from build123d import *

# Parameters (mm, degrees)
EXTRUDE_1_DEPTH      = 10
SKETCH_5_R           = 2.6
CUT_EXTRUDE_3_DEPTH  = 10
FILLET_5_R           = 3
FILLET_6_R           = 3
FILLET_7_R           = 3
SKETCH_7_R           = 5.5
CUT_EXTRUDE_4_DEPTH  = 5
SKETCH_12_R          = 2.553682631
CUT_EXTRUDE_9_DEPTH  = 9
EXTRUDE_2_DEPTH      = 5
CUT_EXTRUDE_START    = 5
SKETCH_14_R          = 5.5
CUT_EXTRUDE_12_DEPTH = 5
EXTRUDE_START        = 5
EXTRUDE_6_DEPTH      = 5
SKETCH_22_R          = 5.5
EXTRUDE_7_DEPTH      = 5
SKETCH_24_R          = 5.5
CUT_EXTRUDE_14_DEPTH = 3
SKETCH_25_R          = 2.65
CUT_EXTRUDE_15_DEPTH = 3
SKETCH_26_R          = 2.65
CUT_EXTRUDE_16_DEPTH = 5
SKETCH_29_R          = 2.65
EXTRUDE_8_DEPTH      = 10
EXTRUDE_START_2      = 3
SKETCH_30_R          = 5.5
EXTRUDE_9_DEPTH      = 3
CUT_EXTRUDE_18_DEPTH = 3
SKETCH_33_R          = 5.5
SKETCH_33_R_2        = 2.6
EXTRUDE_10_DEPTH     = 5
SKETCH_34_W          = 118.655960463
SKETCH_34_H          = 108.474675719
CUT_EXTRUDE_20_DEPTH = 3
CUT_EXTRUDE_21_DEPTH = 108.211729676


with BuildPart() as part:
    # 草图1 → 凸台-拉伸1 (new body)
    with BuildSketch(Plane(origin=(0, 0, 0), x_dir=(1, 0, 0), z_dir=(0, 1, 0))):
        Polygon((0, 0), (0, 80), (80, 0), align=None)
    extrude(amount=EXTRUDE_1_DEPTH)

    # 草图5 → 切除-拉伸3 (cut)
    with BuildSketch(Plane(origin=(0, 10, 0), x_dir=(1, 0, 0), z_dir=(0, 1, 0))):
        with Locations(Location((6.5, 6.5, 0), (0, 0, 270))):
            Circle(SKETCH_5_R)
        with Locations(Location((6.5, 46.5, 0), (0, 0, 270))):
            Circle(SKETCH_5_R)
        with Locations(Location((46.5, 6.5, 0), (0, 0, 270))):
            Circle(SKETCH_5_R)
    extrude(amount=-CUT_EXTRUDE_3_DEPTH, mode=Mode.SUBTRACT)

    # 圆角5
    fillet_5_edges = [part.edges().sort_by_distance(p)[0] for p in [
        (80, 5, 0),
    ]]
    fillet(fillet_5_edges, radius=FILLET_5_R)

    # 圆角6
    fillet_6_edges = [part.edges().sort_by_distance(p)[0] for p in [
        (0, 5, -80),
    ]]
    fillet(fillet_6_edges, radius=FILLET_6_R)

    # 圆角7
    fillet_7_edges = [part.edges().sort_by_distance(p)[0] for p in [
        (0, 5, 0),
    ]]
    fillet(fillet_7_edges, radius=FILLET_7_R)

    # 草图7 → 切除-拉伸4 (cut)
    with BuildSketch(Plane(origin=(0, 10, 0), x_dir=(1, 0, 0), z_dir=(0, 1, 0))):
        with Locations(Location((6.5, 6.5, 0), (0, 0, 270))):
            Circle(SKETCH_7_R)
        with Locations(Location((6.5, 46.5, 0), (0, 0, 270))):
            Circle(SKETCH_7_R)
        with Locations(Location((46.5, 6.5, 0), (0, 0, 270))):
            Circle(SKETCH_7_R)
    extrude(amount=-CUT_EXTRUDE_4_DEPTH, mode=Mode.SUBTRACT)

    # 草图12 → 切除-拉伸9 (cut)
    with BuildSketch(Plane.XZ):
        with Locations((8.5, -46.5)):
            Circle(SKETCH_12_R)
    extrude(amount=-CUT_EXTRUDE_9_DEPTH, mode=Mode.SUBTRACT)

    # 草图13 → 凸台-拉伸2 (add)
    with BuildSketch(Plane.XZ):
        with BuildLine():
            ThreePointArc((7.559676255, -48.87425488), (5.946317369, -46.5), (7.559676255, -44.12574512))
            ThreePointArc((7.559676255, -44.12574512), (3.9, -46.5), (7.559676255, -48.87425488))
        make_face()
    extrude(amount=-EXTRUDE_2_DEPTH)

    # 草图14 → 切除-拉伸12 (cut)
    with BuildSketch(Plane(origin=(0, 5, 0), x_dir=(1, 0, 0), z_dir=(0, 1, 0)).offset(CUT_EXTRUDE_START)):
        with Locations((8.5, 46.5)):
            Circle(SKETCH_14_R)
        with Locations((6.5, 46.5)):
            Circle(SKETCH_14_R)
    extrude(amount=-CUT_EXTRUDE_12_DEPTH, mode=Mode.SUBTRACT)

    # 草图21 → 凸台-拉伸6 (add)
    with BuildSketch(Plane(origin=(0, 5, 0), x_dir=(1, 0, 0), z_dir=(0, 1, 0)).offset(EXTRUDE_START)):
        with BuildLine():
            ThreePointArc((7.5, 41.091673087), (3, 46.5), (7.5, 51.908326913))
            ThreePointArc((7.5, 51.908326913), (1, 46.5), (7.5, 41.091673087))
        make_face()
    extrude(amount=-EXTRUDE_6_DEPTH)

    # 草图22 → 凸台-拉伸7 (add)
    with BuildSketch(Plane(origin=(0, 5, 0), x_dir=(1, 0, 0), z_dir=(0, 1, 0)).offset(EXTRUDE_START)):
        with Locations((8.5, 46.5)):
            Circle(SKETCH_22_R)
    extrude(amount=-EXTRUDE_7_DEPTH)

    # 草图24 → 切除-拉伸14 (cut)
    with BuildSketch(Plane(origin=(0, 10, 0), x_dir=(1, 0, 0), z_dir=(0, 1, 0))):
        with Locations(Location((8.5, 46.5, 0), (0, 0, 270))):
            Circle(SKETCH_24_R)
    extrude(amount=-CUT_EXTRUDE_14_DEPTH, mode=Mode.SUBTRACT)

    # 草图25 → 切除-拉伸15 (cut)
    with BuildSketch(Plane.XZ.offset(-5)):
        with Locations(Location((8.5, -46.5, 0), (0, 0, 270))):
            Circle(SKETCH_25_R)
    extrude(amount=-CUT_EXTRUDE_15_DEPTH, mode=Mode.SUBTRACT)

    # 草图26 → 切除-拉伸16 (cut)
    with BuildSketch(Plane.XZ):
        with Locations(Location((8.5, -46.5, 0), (0, 0, 270))):
            Circle(SKETCH_26_R)
    extrude(amount=-CUT_EXTRUDE_16_DEPTH, mode=Mode.SUBTRACT)

    # 草图29 → 凸台-拉伸8 (add)
    with BuildSketch(Plane.XZ):
        with Locations(Location((8.5, -46.5, 0), (0, 0, 270))):
            Circle(SKETCH_29_R)
    extrude(amount=-EXTRUDE_8_DEPTH)

    # 草图30 → 凸台-拉伸9 (add)
    with BuildSketch(Plane(origin=(0, 7, 0), x_dir=(1, 0, 0), z_dir=(0, 1, 0)).offset(EXTRUDE_START_2)):
        with Locations((8.5, 46.5)):
            Circle(SKETCH_30_R)
    extrude(amount=-EXTRUDE_9_DEPTH)

    # 草图2 → 切除-拉伸18 (cut)
    with BuildSketch(Plane.XZ):
        with BuildLine():
            ThreePointArc((6.5, -56.5), (8.413417162, -56.880602337), (10.035533906, -57.964466094))
            Line((10.035533906, -57.964466094), (57.964466094, -10.035533906))
            ThreePointArc((57.964466094, -10.035533906), (56.880602337, -8.413417162), (56.5, -6.5))
            Line((56.5, -6.5), (54.428932188, -6.5))
            Line((54.428932188, -6.5), (6.5, -54.428932188))
            Line((6.5, -54.428932188), (6.5, -56.5))
        make_face()
        with BuildLine():
            Line((57.964466094, -10.035533906), (10.035533906, -57.964466094))
            ThreePointArc((10.035533906, -57.964466094), (11.119397663, -59.586582838), (11.5, -61.5))
            ThreePointArc((11.5, -61.5), (11.119397663, -63.413417162), (10.035533906, -65.035533906))
            Line((10.035533906, -65.035533906), (65.035533906, -10.035533906))
            ThreePointArc((65.035533906, -10.035533906), (61.5, -11.5), (57.964466094, -10.035533906))
        make_face()
        with BuildLine():
            Line((6.5, -66.5), (6.5, -61.5))
            Line((6.5, -61.5), (6.5, -56.5))
            ThreePointArc((6.5, -56.5), (4.586582838, -56.880602337), (2.964466094, -57.964466094))
            ThreePointArc((2.964466094, -57.964466094), (1.880602337, -63.413417162), (6.5, -66.5))
        make_face()
        with BuildLine():
            Line((6.5, -56.5), (6.5, -61.5))
            Line((6.5, -61.5), (10.035533906, -57.964466094))
            ThreePointArc((10.035533906, -57.964466094), (8.413417162, -56.880602337), (6.5, -56.5))
        make_face()
        with BuildLine():
            Line((10.035533906, -57.964466094), (6.5, -61.5))
            Line((6.5, -61.5), (6.5, -66.5))
            ThreePointArc((6.5, -66.5), (8.413417162, -66.119397663), (10.035533906, -65.035533906))
            ThreePointArc((10.035533906, -65.035533906), (11.119397663, -63.413417162), (11.5, -61.5))
            ThreePointArc((11.5, -61.5), (11.119397663, -59.586582838), (10.035533906, -57.964466094))
        make_face()
        with BuildLine():
            Line((6.5, -56.5), (6.5, -61.5))
            Line((6.5, -61.5), (10.035533906, -57.964466094))
            ThreePointArc((10.035533906, -57.964466094), (8.413417162, -56.880602337), (6.5, -56.5))
        make_face()
        with BuildLine():
            Line((10.035533906, -57.964466094), (6.5, -61.5))
            Line((6.5, -61.5), (6.5, -66.5))
            ThreePointArc((6.5, -66.5), (8.413417162, -66.119397663), (10.035533906, -65.035533906))
            ThreePointArc((10.035533906, -65.035533906), (11.119397663, -63.413417162), (11.5, -61.5))
            ThreePointArc((11.5, -61.5), (11.119397663, -59.586582838), (10.035533906, -57.964466094))
        make_face()
        with BuildLine():
            ThreePointArc((2.964466094, -57.964466094), (4.586582838, -56.880602337), (6.5, -56.5))
            Line((6.5, -56.5), (6.5, -54.428932188))
            Line((6.5, -54.428932188), (2.964466094, -57.964466094))
        make_face()
        with BuildLine():
            Line((54.428932188, -6.5), (56.5, -6.5))
            ThreePointArc((56.5, -6.5), (56.880602337, -4.586582838), (57.964466094, -2.964466094))
            Line((57.964466094, -2.964466094), (54.428932188, -6.5))
        make_face()
        with BuildLine():
            Line((56.5, -6.5), (61.5, -6.5))
            Line((61.5, -6.5), (66.5, -6.5))
            ThreePointArc((66.5, -6.5), (63.413417162, -1.880602337), (57.964466094, -2.964466094))
            ThreePointArc((57.964466094, -2.964466094), (56.880602337, -4.586582838), (56.5, -6.5))
        make_face()
        with BuildLine():
            ThreePointArc((56.5, -6.5), (56.880602337, -8.413417162), (57.964466094, -10.035533906))
            Line((57.964466094, -10.035533906), (61.5, -6.5))
            Line((61.5, -6.5), (56.5, -6.5))
        make_face()
        with BuildLine():
            Line((61.5, -6.5), (57.964466094, -10.035533906))
            ThreePointArc((57.964466094, -10.035533906), (61.5, -11.5), (65.035533906, -10.035533906))
            ThreePointArc((65.035533906, -10.035533906), (66.119397663, -8.413417162), (66.5, -6.5))
            Line((66.5, -6.5), (61.5, -6.5))
        make_face()
        with BuildLine():
            ThreePointArc((56.5, -6.5), (56.880602337, -8.413417162), (57.964466094, -10.035533906))
            Line((57.964466094, -10.035533906), (61.5, -6.5))
            Line((61.5, -6.5), (56.5, -6.5))
        make_face()
        with BuildLine():
            Line((61.5, -6.5), (57.964466094, -10.035533906))
            ThreePointArc((57.964466094, -10.035533906), (61.5, -11.5), (65.035533906, -10.035533906))
            ThreePointArc((65.035533906, -10.035533906), (66.119397663, -8.413417162), (66.5, -6.5))
            Line((66.5, -6.5), (61.5, -6.5))
        make_face()
    extrude(amount=-CUT_EXTRUDE_18_DEPTH, mode=Mode.SUBTRACT)

    # 草图33 → 凸台-拉伸10 (add)
    # profile 1 of 2: a face of its own
    with BuildSketch(Plane(origin=(0, 10, 0), x_dir=(1, 0, 0), z_dir=(0, 1, 0))):
        with Locations((6.5, 6.5)):
            Circle(SKETCH_33_R)
        with Locations(Location((6.5, 6.5, 0), (0, 0, 270))):
            Circle(SKETCH_33_R_2, mode=Mode.SUBTRACT)
    # profile 2 of 2: a face of its own
    with BuildSketch(Plane(origin=(0, 10, 0), x_dir=(1, 0, 0), z_dir=(0, 1, 0))):
        with Locations((46.5, 6.5)):
            Circle(SKETCH_33_R)
        with Locations(Location((46.5, 6.5, 0), (0, 0, 270))):
            Circle(SKETCH_33_R_2, mode=Mode.SUBTRACT)
    extrude(amount=-EXTRUDE_10_DEPTH)

    # 草图34 → 切除-拉伸20 (cut)
    with BuildSketch(Plane(origin=(0, 10, 0), x_dir=(1, 0, 0), z_dir=(0, 1, 0))):
        with Locations((37.4387476, 33.290816779)):
            Rectangle(SKETCH_34_W, SKETCH_34_H)
    extrude(amount=-CUT_EXTRUDE_20_DEPTH, mode=Mode.SUBTRACT)

    # 草图35 → 切除-拉伸21 (cut, through all)
    with BuildSketch(Plane.XZ.offset(-3)):
        with BuildLine():
            Line((8.267766953, -63.267766953), (63.267766953, -8.267766953))
            ThreePointArc((63.267766953, -8.267766953), (63.267766953, -4.732233047), (59.732233047, -4.732233047))
            Line((59.732233047, -4.732233047), (4.732233047, -59.732233047))
            ThreePointArc((4.732233047, -59.732233047), (4.732233047, -63.267766953), (8.267766953, -63.267766953))
        make_face()
    extrude(amount=-CUT_EXTRUDE_21_DEPTH, mode=Mode.SUBTRACT)


solid = part.part
Design review of the part built by this model. Coordinates are the model's own, in mm. A direction names the side the tool comes from. Coordinates: 2 decimals unless noted, no trailing zeros. Write each loop counter-clockwise with the first axis right and the second up, starting at its lowest first coordinate (ties: lowest second). Pieces come first, ordered by that corner, then holes. Notation, with made-up numbers: (60, 66) - (68, 66) arc R28 ccw to (68, 90) - close; hole circle Ø8 at (-10.5, 78.25). An arc over 180 degrees is marked (long way). One line per item, written item: value.
1) Add section B-B (y = 2). State the section outline as (x, z) points.
Answer sheet:
outline: (0, -72.76) arc R3 ccw to (5.12, -74.88) - (74.88, -5.12) arc R3 ccw to (72.76, 0) - (3, 0) arc R3 ccw to (0, -3) - close; hole (2.96, -57.96) arc R5 ccw to (10.04, -65.04) - (65.04, -10.04) arc R5 ccw to (57.96, -2.96) - close; hole circle Ø5.2 at (6.5, -6.5); hole circle Ø5.2 at (46.5, -6.5)
2) Add section D-D (x = 22). State the section outline as (y, z) points, plus the area to 3 significant figures.
Answer sheet:
outline: (0, -58) - (7, -58) - (7, -49.54) - (3, -49.54) - (3, -53.07) - (0, -53.07) - close; (0, -38.93) - (3, -38.93) - (3, -42.46) - (7, -42.46) - (7, 0) - (0, 0) - close
area: 335 mm2
3) Mouldability with a two-part tool opening along Z and no side actions: class faces 4 (the face through (40, 3, -40)), 5 (the face through (4.694, 4.972, -63.228)), 6 (the face through (7.28, 3.55, -4.02)), 7 (the face through (0.86, 3.55, -0.9)) as +Z half, -Z half, draft (parallel to the pull), parting line (faces both ways), or undercut.
Answer sheet:
face 4: -Z half
face 5: undercut
face 6: undercut
face 7: +Z half
4) Insertion check: pin 1 (2 mm diameter, centred on x = 40, y = 3.5, fed in from -Z). The pin has a flat end and moves straight along its axis. Give the tip position at first contact, or say it passes through.
Answer sheet:
pin 1: stops at z = -41
5) For faces 1 (the face through (36, 3, -36)), 2 (the face through (0, 3, -37)), 3 (the face through (35.383, 4.972, -36.153)), list the 3-axis set-ups (+Z, -Z, +X, -X, +Y, -Y) from which the entire face can be reached by the end or side of a thin tool; tool diameter is ignored.
Answer sheet:
face 1: -Y
face 2: +Z, -Z, -X, +Y, -Y
face 3: +Y, -Y
6) Add section C-C (z = -61.5). State the section outline as (x, y) points.
Answer sheet:
outline: (0, 0) - (1.5, 0) - (1.5, 3) - (4, 3) - (4, 7) - (0, 7) - close; (10.04, 3) - (13.57, 3) - (13.57, 0) - (18.5, 0) - (18.5, 7) - (10.04, 7) - close
7) To check wall thickness, follow probe 1 along Z at (x, y) = (46, 1.25); probe 2 along Z at (x, y) = (37.5, 2.5); probe 3 along X at (y, z) = (6.25, -20). State the ranges of each line that lie inside material, in increasing order.
Answer sheet:
probe 1: z = -34 to -29.07, -14.93 to -9.05, -3.95 to 0
probe 2: z = -42.5 to -37.57, -23.43 to 0
probe 3: x = 0 to 44.46, 51.54 to 60
8) Add section A-A (x = 46.5). State the section outline as (y, z) points, plus the area to 3 significant figures.
Answer sheet:
outline: (0, -33.5) - (7, -33.5) - (7, -25.04) - (3, -25.04) - (3, -28.57) - (0, -28.57) - close; (0, -14.43) - (3, -14.43) - (3, -17.96) - (7, -17.96) - (7, -9.1) - (0, -9.1) - close; (0, -3.9) - (7, -3.9) - (7, 0) - (0, 0) - close
area: 127 mm2
